The listing builds one solid part. Answer for the finished solid, in the listing's coordinates (mm). Face numbers are marked on the shaded views. A direction names the side the tool comes from. Give positions to 0.01 mm unless a question says otherwise; leave off trailing zeros. Loops run counter-clockwise (first coordinate to the right, second up) from the corner with the lowest first, then second, coordinate; pieces in that order, holes last. Notation, with made-up numbers: (77.5, 54.25) - (105.5, 54.25) arc R14 ccw to (105.5, 70.25) - close; hole circle Ø3 at (-17.75, -12.75). An arc over 180 degrees is marked (long way). Answer as CSV lines item,"result". Start each with the question number.
1) Flat-ended cylindrical pins translate along their axes: pin 1 (1.9 mm diameter, centred on x = -8.5, z = 9, fed in from -Y); pin 2 (1.8 mm diameter, centred on x = 12.5, z = 5, fed in from -Y); pin 3 (1.7 mm diameter, centred on x = 11, y = 14, fed in from +Z). Find the tip coordinate at first contact, or state that the pin passes through.
2) A cutting plane is placed at C-C (z = 24.5). Determine the outline of the cut face in (x, y).
3) A cutting plane is placed at B-B (y = 13.5). Determine the outline of the cut face in (x, z).
4) A cutting plane is placed at D-D (y = -15). Determine the outline of the cut face in (x, z), and give its area (3 significant figures).
5) A cutting plane is placed at A-A (x = 0). Determine the outline of the cut face in (y, z), and give its area (4 significant figures).
6) For the marked faces 1, 2 and 3, determine the directions among +Z, -Z, +X, -X, +Y, -Y from which every point of the face is accessible in a straight line to the end or side of a thin tool.
7) Find the intervals of material crossed by line 1 along Y through (x, z) = (-14.8, 1.45); line 2 along Z through (x, y) = (-12, -4); line 3 along Y through (x, z) = (-5.5, 12.5), in increasing order.
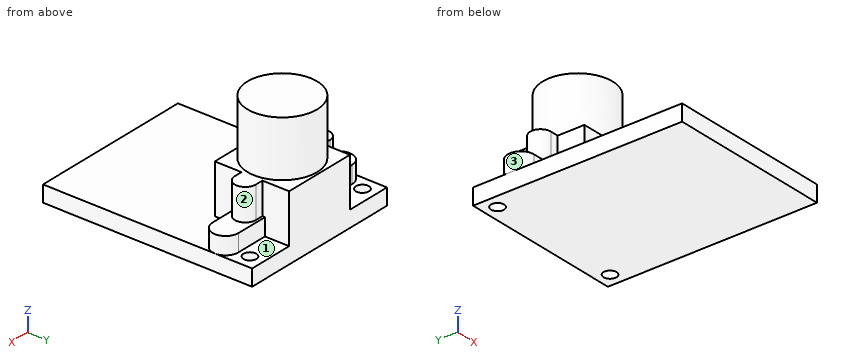
```python
from build123d import *

# Parameters (mm, degrees)
SKETCH_4_W          = 35.5
SKETCH_4_H          = 45
EXTRUDE_2_DEPTH     = 3.5
EXTRUDE_START       = -3.5
SKETCH_5_W          = 16
SKETCH_5_H          = 4.5
SKETCH_5_H_2        = 5.75
EXTRUDE_3_DEPTH     = 14
EXTRUDE_4_DEPTH     = 7.2
EXTRUDE_START_2     = -14
SKETCH_7_R          = 7.5
EXTRUDE_5_DEPTH     = 26
CUT_EXTRUDE_1_REACH = 40.695
SKETCH_8_R          = 1.4


with BuildPart() as part:
    # 草图4 → 凸台-拉伸2 (new body)
    with BuildSketch(Plane.XY):
        Rectangle(SKETCH_4_W, SKETCH_4_H)
    extrude(amount=EXTRUDE_2_DEPTH)

    # 草图5 → 凸台-拉伸3 (add)
    with BuildSketch(Plane.XY.offset(3.5).offset(EXTRUDE_START)):
        with BuildLine():
            Line((-8, 12.25), (-8, 16.75))
            Line((-8, 16.75), (-9.75, 16.75))
            ThreePointArc((-9.75, 16.75), (-12, 14.5), (-9.75, 12.25))
            Line((-9.75, 12.25), (-8, 12.25))
        make_face()
        with Locations((0, 14.5)):
            Rectangle(SKETCH_5_W, SKETCH_5_H)
        with Locations((0, 19.625)):
            Rectangle(SKETCH_5_W, SKETCH_5_H_2)
        with BuildLine():
            Line((9.75, 16.75), (8, 16.75))
            Line((8, 16.75), (8, 12.25))
            Line((8, 12.25), (9.75, 12.25))
            ThreePointArc((9.75, 12.25), (12, 14.5), (9.75, 16.75))
        make_face()
        with Locations((0, 9.375)):
            Rectangle(SKETCH_5_W, SKETCH_5_H_2)
    extrude(amount=EXTRUDE_3_DEPTH)

    # 草图6 → 凸台-拉伸4 (add)
    with BuildSketch(Plane.XY.offset(3.5).offset(EXTRUDE_START)):
        with BuildLine():
            Line((-14.95, 17.3), (14.95, 17.3))
            ThreePointArc((14.95, 17.3), (17.75, 14.5), (14.95, 11.7))
            Line((14.95, 11.7), (-14.95, 11.7))
            ThreePointArc((-14.95, 11.7), (-17.75, 14.5), (-14.95, 17.3))
        make_face()
    extrude(amount=EXTRUDE_4_DEPTH)

    # 草图7 → 凸台-拉伸5 (add)
    with BuildSketch(Plane.XY.offset(14).offset(EXTRUDE_START_2)):
        with Locations(Location((0, 14.5, 0), (0, 0, 180))):
            Circle(SKETCH_7_R)
    extrude(amount=EXTRUDE_5_DEPTH)

    # 草图8 → 切除-拉伸1 (cut, up to next)
    with BuildSketch(Plane(origin=(0, 0, 0), x_dir=(-1, 0, 0), z_dir=(0, 0, -1)), mode=Mode.PRIVATE) as cut_extrude_1_sk1:
        with Locations((-14.8, 19.626575336)):
            Circle(SKETCH_8_R)
    cut_extrude_1_tool1 = extrude(cut_extrude_1_sk1.sketch, amount=-CUT_EXTRUDE_1_REACH, mode=Mode.PRIVATE) & part.part
    # 草图8 → 切除-拉伸1 (cut, up to next)
    with BuildSketch(Plane(origin=(0, 0, 0), x_dir=(-1, 0, 0), z_dir=(0, 0, -1)), mode=Mode.PRIVATE) as cut_extrude_1_sk2:
        with Locations(Location((14.8, 19.626575336, 0), (0, 0, 180))):
            Circle(SKETCH_8_R)
    cut_extrude_1_tool2 = extrude(cut_extrude_1_sk2.sketch, amount=-CUT_EXTRUDE_1_REACH, mode=Mode.PRIVATE) & part.part
    add(cut_extrude_1_tool1.solids().sort_by_distance((14.8, 19.626575, 0))[0], mode=Mode.SUBTRACT)
    add(cut_extrude_1_tool2.solids().sort_by_distance((-14.8, 19.626575, 0))[0], mode=Mode.SUBTRACT)


solid = part.part
```
Ans:
1,pin 1,"y = 6.5"
1,pin 2,"y = 11.7"
1,pin 3,"z = 14"
2,outline,"circle Ø15 at (0, 14.5)"
3,outline,"(-17.75, 0) - (17.75, 0) - (17.75, 3.5) - (17.57, 3.5) - (17.57, 7.2) - (11.77, 7.2) - (11.77, 14) - (7.43, 14) - (7.43, 26) - (-7.43, 26) - (-7.43, 14) - (-11.77, 14) - (-11.77, 7.2) - (-17.57, 7.2) - (-17.57, 3.5) - (-17.75, 3.5) - close"
4,outline,"(-17.75, 0) - (17.75, 0) - (17.75, 3.5) - (-17.75, 3.5) - close"
4,area,"124 mm2"
5,outline,"(-22.5, 0) - (22.5, 0) - (22.5, 14) - (22, 14) - (22, 26) - (7, 26) - (7, 14) - (6.5, 14) - (6.5, 3.5) - (-22.5, 3.5) - close"
5,area,"505.5 mm2"
6,face 1,"+Z, +X, +Y"
6,face 2,"+Z, +X"
6,face 3,"+Z, -X"
7,line 1,"-22.5 to 18.23, 21.03 to 22.5"
7,line 2,"0 to 3.5"
7,line 3,"6.5 to 22.5"
